```python
from build123d import *

# Parameters (mm, degrees)
F1_DEPTH       = 22.352
F3_DEPTH       = 79.502
F6_D           = 19.05
F6_DEPTH       = 12.7
F6_START       = 57.15
F6_CBORE_D     = 38.1
F6_CBORE_DEPTH = 3.048
F6_TIP         = 5.7231973962
F8_D           = 19.05
F8_CSINK_D     = 38.1
F8_CSINK_ANGLE = 82
F9_R           = 15.748


with BuildPart() as f1:
    # F0 (on Top) → F1 (new body)
    with BuildSketch(Plane.XY):
        with BuildLine():
            Line((91.948, 127), (72.898, 127))
            Line((72.898, 127), (72.898, 107.95))
            ThreePointArc((72.898, 107.95), (78.4776158184, 121.4203841816), (91.948, 127))
        make_face()
        with BuildLine():
            Line((72.898, 19.05), (72.898, 0))
            Line((72.898, 0), (91.948, 0))
            ThreePointArc((91.948, 0), (78.4776158184, 5.5796158184), (72.898, 19.05))
        make_face()
        Polygon((0, 127), (0, 0), (72.898, 0), (72.898, 19.05), (72.898, 107.95), (72.898, 127), align=None)
    extrude(amount=F1_DEPTH)

    # F2 (on face) → F3 (join)
    with BuildSketch(Plane.XY):
        with BuildLine():
            Line((72.898, 107.95), (72.898, 19.05))
            ThreePointArc((72.898, 19.05), (78.4776158184, 5.5796158184), (91.948, 0))
            Line((91.948, 0), (241.3, 0))
            Line((241.3, 0), (241.3, 127))
            Line((241.3, 127), (91.948, 127))
            ThreePointArc((91.948, 127), (78.4776158184, 121.4203841816), (72.898, 107.95))
        make_face()
    extrude(amount=F3_DEPTH)

    # F6
    # its depths count from where the whole tool has entered the part; down to there all is cleared
    with Locations(Plane.XY.offset(79.502)):
        with Locations((35.052, 95.25)):
            Hole(F6_CBORE_D / 2, depth=F6_START)
    with Locations(Plane.XY.offset(79.502)):
        with Locations((199.898, 35.052, 0), (35.052, 95.25, -F6_START)):
            CounterBoreHole(F6_D / 2, F6_CBORE_D / 2, F6_CBORE_DEPTH, depth=F6_DEPTH)
            with Locations((0, 0, -(F6_DEPTH + F6_TIP / 2))):  # 118° drill point
                Cone(0, F6_D / 2, F6_TIP, mode=Mode.SUBTRACT)

    # F8 (through all)
    with Locations(Plane.XY.offset(79.502)):
        with Locations((152.4, 95.25), (114.3, 35.052)):
            CounterSinkHole(F8_D / 2, F8_CSINK_D / 2, counter_sink_angle=F8_CSINK_ANGLE)

    # F9
    f9_edges = [f1.edges().sort_by_distance(p)[0] for p in [
        (0, 0, 11.176),
        (0, 127, 11.176),
        (241.3, 0, 39.751),
        (241.3, 127, 39.751),
    ]]
    fillet(f9_edges, radius=F9_R)


solid = f1.part
```
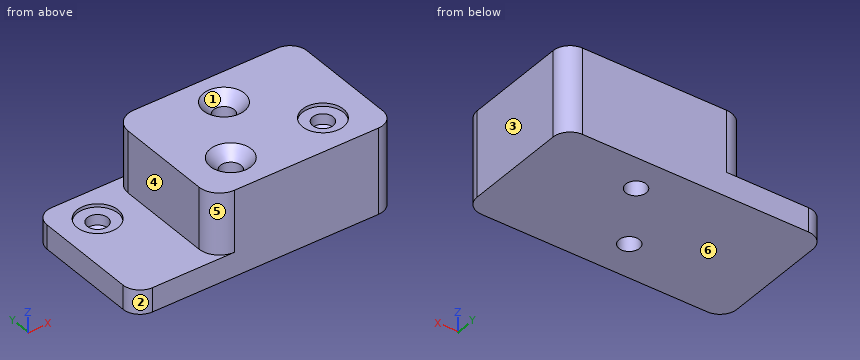
For this review, take the finished solid that the model builds, in its own axes (mm). Face numbers are marked on the shaded views. A direction names the side the tool comes from. Round coordinates to 2 decimals unless told otherwise and drop trailing zeros. Write each loop counter-clockwise with the first axis right and the second up, starting at its lowest first coordinate (ties: lowest second). Pieces come first, ordered by that corner, then holes. Notation, with made-up numbers: M 60,45.25 L 82,45.25 A16 cw 82,69.25 Z; hole C 31,-39 d9. An arc over 180 degrees is marked long. One line per item, written item: value. Start each with the question number.
(1) The part is to be moulded in two halves that separate along Y. For the marked faces 1, 2 and 3, say which applies: released by +Y, released by -Y, zero draft, split by the parting line, or undercut.
(2) Insertion check: pin 1 (6 mm diameter, centred on y = 82, z = 45.5, fed in from -X); pin 2 (25 mm diameter, centred on x = 114.3, y = 35.052, fed in from +Z); pin 3 (23 mm diameter, centred on x = 199.898, y = 35.052, fed in from +Z). Each pin has a flat end and moves straight along its axis. Give the tip position at first contact, or say it passes through.
(3) Wall thickness on line 1 (X direction, y = 95.25, z = 27) (3 decimals); line 2 (X direction, y = 38, z = 67); line 3 (Y direction, x = 114, z = 17): over which ranges is each line inside the solid? List them lowest first.
(4) We need section C-C (z = 73). Give the boundary of the cut face in (x, y) (3 decimals).
(5) We need section D-D (y = 12). Give the boundary of the cut face in (x, z), and give its area (3 significant figures).
(6) We need section B-B (z = 36.5). Give the boundary of the cut face in (x, y) (3 decimals).
(7) We need section A-A (x = 152.4). Give the boundary of the cut face in (y, z) (3 decimals), and give its area (3 significant figures).
(8) Machinability: for the marked faces 4, 5 and 6, which of the approach directions +Z, -Z, +X, -X, +Y, -Y give a long, thin tool a straight path to every point of the face, cutting with its end or side? Answer none if there is none.
Result:
1. face 1: undercut
1. face 2: released by -Y
1. face 3: zero draft
2. pin 1: x = 72.9
2. pin 2: z = 71.97
2. pin 3: z = 76.45
3. line 1: 72.898 to 142.875, 161.925 to 241.3
3. line 2: 72.9 to 105.24, 123.36 to 190.84, 208.96 to 241.3
3. line 3: 0 to 25.53, 44.57 to 127
4. outline: M 72.898,19.05 A19.05 ccw 91.948,0 L 225.552,0 A15.748 ccw 241.3,15.748 L 241.3,111.252 A15.748 ccw 225.552,127 L 91.948,127 A19.05 ccw 72.898,107.95 Z; hole C 114.3,35.052 d26.796; hole C 152.4,95.25 d26.796; hole C 199.898,35.052 d19.05
5. outline: M 0.45,0 L 240.85,0 L 240.85,79.5 L 74.25,79.5 L 74.25,22.35 L 0.45,22.35 Z
5. area: 14,900 mm²
6. outline: M 72.898,19.05 A19.05 ccw 91.948,0 L 225.552,0 A15.748 ccw 241.3,15.748 L 241.3,111.252 A15.748 ccw 225.552,127 L 91.948,127 A19.05 ccw 72.898,107.95 Z; hole C 114.3,35.052 d19.05; hole C 152.4,95.25 d19.05
7. outline: M 0,0 L 85.725,0 L 85.725,68.545 L 76.2,79.502 L 0,79.502 Z; M 104.775,0 L 127,0 L 127,79.502 L 114.3,79.502 L 104.775,68.545 Z
7. area: 8,480 mm²
8. face 4: +Z, -X, +Y, -Y
8. face 5: +Z, -X, -Y
8. face 6: -Z, +X, -X, +Y, -Y
